Source: CAD feature listing. Evaluate the final solid. Frame: model axes, mm. A direction names the side the tool comes from. Give positions to 0.01 mm unless a question says otherwise; leave off trailing zeros. Loops run counter-clockwise (first coordinate to the right, second up) from the corner with the lowest first, then second, coordinate; pieces in that order, holes last. Notation, with made-up numbers: M -39.5,28 L -33.5,28 A28 cw -33.5,56 Z; hole C 82,70.5 d9. An arc over 180 degrees is marked long. Answer in a Markdown table with one row per item.
```python
from build123d import *

# Parameters (mm, degrees)
SM_BASE_FLANGE_1_DEPTH = 3
OTHER_START            = -10
OTHER_1_DEPTH          = 20
OTHER_1_2_DEPTH        = 20
CUT_EXTRUDE_1_DEPTH    = 55.411051267
FILLET_1_R             = 2


# Read off the part's stored shape, not the designer's step: 转折1
# Sheet-metal steps are written as plain solids
with BuildPart() as part:
    # Sketch 2 → 基体-法兰1 (new body)
    with BuildSketch(Plane(origin=(0, 0, 0), x_dir=(1, 0, 0), z_dir=(0, 1, 0))):
        with BuildLine():
            Line((-12.031587919, -10), (-7.7014609, -7.5))
            ThreePointArc((-7.7014609, -7.5), (10.75, 0), (-7.7014609, 7.5))
            Line((-7.7014609, 7.5), (-12.031587919, 10))
            Line((-12.031587919, 10), (-53, 10))
            Line((-53, 10), (-53, -10))
            Line((-53, -10), (-12.031587919, -10))
        make_face()
    extrude(amount=-SM_BASE_FLANGE_1_DEPTH)

    # Other 1 outline → Other 1 (cut)
    with BuildSketch(Plane.XY.offset(OTHER_START)):
        with BuildLine():
            ThreePointArc((-18.007123317, -3), (-18.981991132, -2.871656217), (-19.890423317, -2.495371286))
            Line((-19.890423317, -2.495371286), (-24.212533168, 0))
            Line((-24.212533168, 0), (-53, 0))
            Line((-53, 0), (-53, -3))
            Line((-53, -3), (-18.007123317, -3))
        make_face()
    extrude(amount=OTHER_1_DEPTH, mode=Mode.SUBTRACT)

    # Other 1 2 outline → Other 1 2 (add)
    with BuildSketch(Plane.XY.offset(OTHER_START)):
        with BuildLine():
            Line((-29.230795442, 2.897295075), (-24.212533168, 0))
            Line((-24.212533168, 0), (-18.007123317, 0))
            ThreePointArc((-18.007123317, 0), (-18.205533997, 0.026121262), (-18.390423317, 0.102704925))
            Line((-18.390423317, 0.102704925), (-27.730795442, 5.495371286))
            ThreePointArc((-27.730795442, 5.495371286), (-28.639227627, 5.871656217), (-29.614095442, 6))
            Line((-29.614095442, 6), (-53, 6))
            Line((-53, 6), (-53, 3))
            Line((-53, 3), (-29.614095442, 3))
            ThreePointArc((-29.614095442, 3), (-29.415684762, 2.973878738), (-29.230795442, 2.897295075))
        make_face()
    extrude(amount=OTHER_1_2_DEPTH)

    # 草图8 → 切除-拉伸1 (cut, through all)
    with BuildSketch(Plane(origin=(0, 0, 0), x_dir=(1, 0, 0), z_dir=(0, 1, 0))):
        Polygon((0, 7.071067812), (-7.071067812, 0), (0, -7.071067812), (7.071067812, 0), align=None)
    extrude(amount=-CUT_EXTRUDE_1_DEPTH, mode=Mode.SUBTRACT)

    # 圆角1
    fillet_1_edges = [part.edges().sort_by_distance(p)[0] for p in [
        (-53, 4.5, 10),
        (-53, 4.5, -10),
    ]]
    fillet(fillet_1_edges, radius=FILLET_1_R)


solid = part.part
```
Q1. Section query A-A (z = -2.5). Output: boundary loops of the cut face in (x, y).
Values follow:
| item | result |
|---|---|
| outline | M -53,3 L -29.61,3 A0.77 cw -29.23,2.9 L -19.89,-2.5 A3.77 ccw -18.01,-3 L -4.57,-3 L -4.57,0 L -18.01,0 A0.77 cw -18.39,0.1 L -27.73,5.5 A3.77 ccw -29.61,6 L -53,6 Z; M 4.57,-3 L 10.46,-3 L 10.46,0 L 4.57,0 Z |
Q2. Ray query, probe 1 along Z at (x, y) = (-28, 4.5); probe 2 along Y at (x, z) = (-12, 1); probe 3 along Y at (x, z) = (-49, 5.5). Return the intervals inside material, ascending. Write a range as from..to.
Values follow:
| item | result |
|---|---|
| probe 1 | -10..10 |
| probe 2 | -3..0 |
| probe 3 | 3..6 |
Q3. Reachability of faces 1 (the flat face through (-9.836, -1.479, -8.732)), 2 (the flat face through (3.585, -1.479, -3.486)), 3 (the flat face through (-32, 4, -10)), 4 (the flat face through (-32, 4, 10)) from +Z, -Z, +X, -X, +Y, -Y: full face, straight path, thin tool, end or side. Return the list, or none.
Values follow:
| item | result |
|---|---|
| face 1 | -Z, +Y, -Y |
| face 2 | +Y, -Y |
| face 3 | -Z, -X, +Y, -Y |
| face 4 | +Z, -X, +Y, -Y |
Q4. Contact query for flat-ended pins moving along their axis: pin 1 Ø4.5 at (x, y) = (-22.5, 0.5) entering from -Z; pin 2 Ø10.5 at (x, z) = (-2, 2) entering from +Y; pin 3 Ø2 at (y, z) = (0, 6.5) entering from -X. Output: stop coordinate, or through.
Values follow:
| item | result |
|---|---|
| pin 1 | z = -10 |
| pin 2 | y = 0 |
| pin 3 | x = -25.94 |
Q5. Section query B-B (x = -13.5). Output: boundary loops of the cut face in (y, z), plus the area to 3 significant figures.
Values follow:
| item | result |
|---|---|
| outline | M -3,-10 L 0,-10 L 0,10 L -3,10 Z |
| area | 60.0 mm^2 |
Q6. Mould query, pull axis Z, two halves, no side actions, for faces 5 (the flat face through (-41, 3, 0)), 6 (the flat face through (-9.9, -1.48, 8.77)), 7 (the flat face through (-3.486, -1.479, -3.585)). Classes: +Z half, -Z half, draft (parallel to the pull), parting line (faces both ways), or undercut.
Values follow:
| item | result |
|---|---|
| face 5 | draft |
| face 6 | +Z half |
| face 7 | undercut |
Q7. Section query D-D (y = 2). Output: boundary loops of the cut face in (x, z).
Values follow:
| item | result |
|---|---|
| outline | M -27.68,-10 L -21.68,-10 L -21.68,10 L -27.68,10 Z |
Q8. Section query C-C (z = 1). Output: boundary loops of the cut face in (x, y).
Values follow:
| item | result |
|---|---|
| outline | M -53,3 L -29.61,3 A0.77 cw -29.23,2.9 L -19.89,-2.5 A3.77 ccw -18.01,-3 L -6.07,-3 L -6.07,0 L -18.01,0 A0.77 cw -18.39,0.1 L -27.73,5.5 A3.77 ccw -29.61,6 L -53,6 Z; M 6.07,-3 L 10.7,-3 L 10.7,0 L 6.07,0 Z |
